Input: part model. Units: mm. Frame: model coordinates. A direction names the side the tool comes from. Round coordinates to 2 decimals unless told otherwise and drop trailing zeros. Loops run counter-clockwise (first coordinate to the right, second up) from the corner with the lowest first, then second, coordinate; pieces in that order, holes last.
(1) Cut plane A-A, the plane y = 3.55. Output: boundary loops of the cut face in (x, z) (3 decimals).
(2) Access query for faces 1 (the face through (10, 3, -22.213)), 2 (the face through (20.425, 3.974, -45.107)), 3 (the face through (20.3, 4.775, -45.5)). Directions: +Z, -Z, +X, -X, +Y, -Y. A direction counts if a zero-diameter tool reaches every point of the face in a straight line with its end or side. Return the directions, or none.
(3) Draft query along Z for faces 4 (the face through (12, 3, -21.288)), 5 (the face through (21, 1.51, -44)), 6 (the face through (21.4, 3.15, -45.8)). Return one class per face: released by +Z, released by -Z, zero draft, split by the parting line, or undercut.
(4) Line query: line 1 (X direction, y = 1.7, z = -45); line 2 (X direction, y = 2.55, z = -49); line 3 (Z direction, x = 20.5, y = 2.65). Output: solid intervals per line, ascending.
(5) First-contact query: pin 1 Ø1.5 at (y, z) = (3, -26.5) entering from -X; pin 2 Ø1 at (x, y) = (32.5, 3) entering from +Z; pin 3 Ø16.5 at (x, z) = (25, -35) entering from +Y (3 decimals); pin 4 Ø1 at (x, y) = (10.5, 3.5) entering from +Z. Flat tips, straight axial feed; report the tip coordinate or a pass-through.
(6) Cut plane C-C, the plane z = -52. Output: boundary loops of the cut face in (x, y) (3 decimals), and give its area (3 significant figures).
(7) Cut plane B-B, the plane x = 31.5. Output: boundary loops of the cut face in (y, z) (3 decimals), and give its area (3 significant figures).
from build123d import *

# Parameters (mm, degrees)
SKETCH1_W          = 2.06
SKETCH1_H          = 6.53
SKETCH3_W          = 1.5
SKETCH3_H          = 6.53
SKETCH6_W          = 2.34
SKETCH6_H          = 6.53
CUT_EXTRUDE1_DEPTH = 3.25
SCALE1_SCALE       = 0.5


with BuildPart() as part:
    # Sweep1: sweep along a path in Sketch2
    with BuildLine(Plane(origin=(0, 0, 0), x_dir=(1, 0, 0), z_dir=(0, 1, 0))) as sweep1_path:
        ThreePointArc((2.06, 0), (20.505721927, 44.951087367), (65.415754098, 63.496542965))
    # Sketch1 → Sweep1 (sweep)
    with BuildSketch(Plane.XY):
        with Locations((1.03, 3.265)):
            Rectangle(SKETCH1_W, SKETCH1_H)
    sweep(path=sweep1_path.line)

    # Sweep2: sweep along a path in Sketch4
    with BuildLine(Plane(origin=(0, 0, 0), x_dir=(1, 0, 0), z_dir=(0, 1, 0))) as sweep2_path:
        ThreePointArc((-2.34, 1.85), (17.612800495, 48.600532533), (64.642950035, 67.885023038))
    # Sketch3 → Sweep2 (sweep)
    with BuildSketch(Plane.XY.offset(-1.85)):
        with Locations((-0.75, 3.265)):
            Rectangle(SKETCH3_W, SKETCH3_H)
    sweep(path=sweep2_path.line)

    # Sweep3: sweep along a path in Sketch7
    with BuildLine(Plane(origin=(0, 6.53, 0), x_dir=(1, 0, 0), z_dir=(0, 1, 0))) as sweep3_path:
        ThreePointArc((-1.5, 1.85), (18.444326424, 47.774036761), (64.654921624, 67.045108351))
    # Sketch6 → Sweep3 (sweep)
    with BuildSketch(Plane.XY.offset(-1.85)):
        with Locations((-2.67, 3.265)):
            Rectangle(SKETCH6_W, SKETCH6_H)
    sweep(path=sweep3_path.line)

    # Sketch8 → Cut-Extrude1 (cut)
    with BuildSketch(Plane(origin=(0, 6.53, 0), x_dir=(1, 0, 0), z_dir=(0, 1, 0))):
        with BuildLine():
            Line((0, 1.85), (-1.4905859, 1.85))
            ThreePointArc((-1.4905859, 1.85), (18.079818822, 48.146737329), (64.654921624, 67.045108351))
            Line((64.654921624, 67.045108351), (64.676165293, 65.554673837))
            ThreePointArc((64.676165293, 65.554673837), (19.144412702, 47.097209332), (0, 1.85))
        make_face()
    extrude(amount=-CUT_EXTRUDE1_DEPTH, mode=Mode.SUBTRACT)


with BuildPart() as part_1:
    # Scale1: scaled about (23.281504141, 3.019990998, -42.576303798)
    add(part.part.scale(SCALE1_SCALE).moved(Location((11.64075207, 1.509995499, -21.288151899))))


solid = part_1.part
Reported:
1. outline: (9.721, -22.213) arc R34.664 ccw to (43.923, -55.98) - (43.968, -54.811) arc R32.836 cw to (10.895, -22.213) - close; (11.641, -22.213) arc R32.096 ccw to (43.979, -54.065) arc R32.605 ccw to (44.358, -54.066) - (44.349, -53.036) arc R31.575 cw to (12.671, -21.288) - (11.641, -21.288) arc R32.605 ccw to (43.433, -54.056) arc R32.325 cw to start
2. face 1: +Z, -X, +Y, -Y
2. face 2: +Y
2. face 3: +Z, -Z, +X, -X, +Y
3. face 4: released by +Z
3. face 5: zero draft
3. face 6: undercut
4. line 1: x = 19.06 to 21.52, 21.68 to 23.2
4. line 2: x = 23.51 to 26.6, 26.79 to 28.8
4. line 3: z = -46.45 to -43.97, -43.81 to -42.27
5. pin 1: stops at x = 9.99
5. pin 2: stops at z = -50.57
5. pin 3: stops at y = 4.775
5. pin 4: stops at z = -22.21
6. outline: (28.241, 1.51) - (32.605, 1.51) - (32.605, 4.775) - (32.406, 4.775) - (32.406, 3.15) - (30.436, 3.15) - (30.436, 4.775) - (28.241, 4.775) - close; (32.822, 1.51) - (36.221, 1.51) - (36.221, 4.775) - (32.822, 4.775) - close
6. area: 22.1 mm2
7. outline: (1.51, -53.504) - (4.775, -53.504) - (4.775, -52.449) - (3.15, -52.449) - (3.15, -51.643) - (4.775, -51.643) - (4.775, -51.562) - (1.51, -51.562) - close; (1.51, -51.472) - (4.775, -51.472) - (4.775, -50.35) - (1.51, -50.35) - close
7. area: 8.69 mm2
